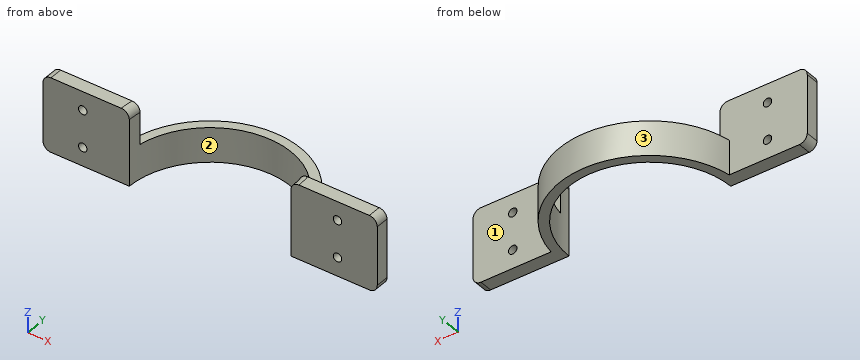
Autodesk Inventor part; units mm, degrees
ref_plane "YZ Plane" through (0, 0, 0) normal (1, 0, 0) x (0, 1, 0)
ref_plane "XZ Plane" through (0, 0, 0) normal (0, 1, 0) x (-1, 0, 0)
ref_plane "XY Plane" through (0, 0, 0) normal (0, 0, 1) x (1, 0, 0)
sketch "Эскиз1" plane through (0, 0, 0) normal (0, 0, 1) x (1, 0, 0)
  circle A0 centre (0, 0) radius 30.5
  circle A1 centre (0, 0) radius 34
  line L0 (0, 0) -> (-48.0635, 0)
  line L1 (-48.0635, 0) -> (48.0635, 0)
  line L2 (-48.0635, 0) -> (-63.0635, 0)
  line L3 (48.0635, 0) -> (63.0635, 0)
  line L4 (-63.0635, 0) -> (-63.0635, 5)
  line L5 (-63.0635, 5) -> (48.0635, 5)
  line L6 (48.0635, 5) -> (48.0635, 0)
  line L7 (63.0635, 0) -> (63.0635, 5)
  line L8 (63.0635, 5) -> (48.0635, 5)
  point P0 (-30.5, 0)
  point P1 (30.5, 0)
  point P2 (34, 0)
  point P3 (-34, 0)
  point P4 (33.6303, 5)
  point P5 (-33.6303, 5)
  dimension "d0" = 61
  dimension "d1" = 68
  dimension "d2" = 48.0635
  dimension "d3" = 96.127
  dimension "d4" = 15
  dimension "d5" = 15
  dimension "d9" = 5
extrude "Выдавливание1" add sketch "Эскиз1" along normal blind 13 contours A0 L5 A1 L1 | A0 L5 A1 | L0 A1 L5 A0 | A1 L5 L6 L1 | L0 L2 L4 L5 A1 | L6 L8 L7 L3
sketch "Эскиз2" plane through (0, 0, 13) normal (0, 0, 1) x (1, 0, 0)
  circle A0 centre (0, 0) radius 30.5
  line L0 (-63.0635, 0) -> (-30.5, 0)
  line L1 (-63.0635, 0) -> (-30.0874, 0)
  line L2 (-30.0874, 0) -> (-30.0874, 5)
  line L3 (-30.0874, 5) -> (-63.0635, 5)
  line L4 (-63.0635, 5) -> (-63.0635, 0)
  line L5 (30.5, 0) -> (63.0635, 0)
  arc A1 (30.5, 0) -> (-30.5, 0) centre (0, 0) ccw
  line L6 (63.0635, 0) -> (30.0874, 0)
  line L7 (30.0874, 0) -> (30.0874, 5)
  line L8 (30.0874, 5) -> (63.0635, 5)
  line L9 (63.0635, 5) -> (63.0635, 0)
extrude "Выдавливание2" add sketch "Эскиз2" along normal blind 15 contours A0 L8 L9 L5 | L0 L4 L3 A0
sketch "Эскиз3" plane through (-63.0635, 5, 0) normal (0, 1, 0) x (1, 0, 0)
  line L0 (0, 0) -> (32.5635, 0)
  line L1 (0, 0) -> (15, 0)
  line L2 (15, 0) -> (15, -7)
  line L3 (15, -7) -> (15, -21)
  line L4 (93.5635, 0) -> (126.127, 0)
  line L5 (126.127, 0) -> (111.127, 0)
  line L6 (111.127, 0) -> (111.127, -7)
  line L7 (111.127, -7) -> (111.127, -21)
  circle A0 centre (111.127, -21) radius 1.6
  circle A1 centre (111.127, -7) radius 1.6
  circle A2 centre (15, -21) radius 1.6
  circle A3 centre (15, -7) radius 1.6
  point P0 (63.0635, 0)
  dimension "d12" = 15
  dimension "d13" = 7
  dimension "d14" = 14
  dimension "d15" = 15
  dimension "d16" = 3.2
  dimension "d17" = 3.2
  dimension "d18" = 3.2
  dimension "d19" = 3.2
extrude "Выдавливание3" cut sketch "Эскиз3" against normal blind 15
fillet "Сопряжение1" radius 3 6 edges at (30.3967, 2.5085, 28) (63.0635, 2.5, 28) (63.0635, 2.5, 0) (-63.0635, 2.5, 0) (-63.0635, 2.5, 28) (-30.3967, 2.5085, 28)
properties part number "vydacha_2"
CAD build for the part. Positions are in the model's coordinates, mm. Face numbers are marked on the shaded views. Round coordinates to 2 decimals unless told otherwise and drop trailing zeros. Order: outer loops, then holes, each group sorted by start corner. A loop starts at its lowest first (then second) coordinate and runs counter-clockwise, first axis right, second up. Notation, with made-up numbers: (-2, 18.25) - (2, 18.25) arc R12 ccw to (2, 41.25) - close; hole circle Ø3 at (47, 33). An arc over 180 degrees is marked (long way). Return JSON: item names as keys, results as strings.
(1) Cut at A-A (z = 21). Give the cut face in (x, y).
Answer key:
{"outline": "(-63.06, 0) - (-49.66, 0) - (-49.66, 5) - (-63.06, 5) - close; (-46.46, 0) - (-30.5, 0) arc R30.5 cw to (-30.09, 5) - (-46.46, 5) - close; (30.09, 5) arc R30.5 cw to (30.5, 0) - (46.46, 0) - (46.46, 5) - close; (49.66, 0) - (63.06, 0) - (63.06, 5) - (49.66, 5) - close"}
(2) Wall check: probe 1 along X at (y, z) = (3.8, 21); probe 2 along X at (y, z) = (1.25, 21); probe 3 along Y at (x, z) = (-5, 7.75). Give the ranges that are in metal, low to high. Write a range as from..to.
Answer key:
{"probe 1": "x = -63.06..-49.66, -46.46..-30.26, 30.26..46.46, 49.66..63.06", "probe 2": "x = -63.06..-49.66, -46.46..-30.47, 30.47..46.46, 49.66..63.06", "probe 3": "y = 30.09..33.63"}
(3) Cut at B-B (y = 16.5). Give the cut face in (x, z).
Answer key:
{"outline": "(-29.73, 0) - (-25.65, 0) - (-25.65, 13) - (-29.73, 13) - close; (25.65, 0) - (29.73, 0) - (29.73, 13) - (25.65, 13) - close"}
(4) Pin check, flat tips, straight feed: pin 1 Ø8.5 at (x, z) = (48, 7.5) entering from +Y; pin 2 Ø8 at (y, z) = (30, 6) entering from -X; pin 3 Ø10 at (x, z) = (-8.5, 8) entering from -Y; pin 4 Ø1.9 at (x, z) = (-48.06, 7) entering from -Y. Stop position of each tip, or through.
Answer key:
{"pin 1": "stops at y = 5", "pin 2": "stops at x = -21.91", "pin 3": "stops at y = 27.35", "pin 4": "passes through"}
(5) Pull direction X, two halves, no side cores. Call the marked faces 1, 2 and 3: +X half, -X half, draft (parallel to the pull), parting line (faces both ways), or undercut.
Answer key:
{"face 1": "draft", "face 2": "undercut", "face 3": "parting line"}
(6) Cut at D-D (x = 0). Give the cut face in (y, z).
Answer key:
{"outline": "(30.5, 0) - (34, 0) - (34, 13) - (30.5, 13) - close"}
(7) Cut at C-C (x = -44). Give the cut face in (y, z), then the cut area to 3 significant figures.
Answer key:
{"outline": "(0, 0) - (5, 0) - (5, 28) - (0, 28) - close", "area": "140 mm^2"}
